from build123d import *

# Parameters (mm, degrees)
SKETCH1_W           = 24.7
SKETCH1_H           = 6.85
SKETCH1_R           = 1.4
BOSS_EXTRUDE1_DEPTH = 0.8
CHAMFER1_SIZE       = 1
SKETCH2_R           = 2
SKETCH2_R_2         = 1.4
BOSS_EXTRUDE2_DEPTH = 0.01


with BuildPart() as part:
    # Sketch1 → Boss-Extrude1 (new body, symmetric)
    with BuildSketch(Plane(origin=(0, 0, 0), x_dir=(1, 0, 0), z_dir=(0, 1, 0))):
        Rectangle(SKETCH1_W, SKETCH1_H)
        with Locations((-2.5, 0)):
            Circle(SKETCH1_R, mode=Mode.SUBTRACT)
        with Locations((2.5, 0)):
            Circle(SKETCH1_R, mode=Mode.SUBTRACT)
        with BuildLine():
            Line((-10.2, 1.25), (-6.8, 1.25))
            ThreePointArc((-6.8, 1.25), (-5.55, 0), (-6.8, -1.25))
            Line((-6.8, -1.25), (-10.2, -1.25))
            ThreePointArc((-10.2, -1.25), (-11.45, 0), (-10.2, 1.25))
        make_face(mode=Mode.SUBTRACT)
        with BuildLine():
            Line((10.2, 1.25), (6.8, 1.25))
            ThreePointArc((6.8, 1.25), (5.55, 0), (6.8, -1.25))
            Line((6.8, -1.25), (10.2, -1.25))
            ThreePointArc((10.2, -1.25), (11.45, 0), (10.2, 1.25))
        make_face(mode=Mode.SUBTRACT)
    extrude(amount=BOSS_EXTRUDE1_DEPTH, both=True)

    # Chamfer1
    chamfer1_edges = [part.edges().sort_by_distance(p)[0] for p in [
        (12.35, 0, 3.425),
        (-12.35, 0, 3.425),
        (-12.35, 0, -3.425),
        (12.35, 0, -3.425),
    ]]
    chamfer(chamfer1_edges, length=CHAMFER1_SIZE)

    # Sketch2 → Boss-Extrude2 (add)
    with BuildSketch(Plane(origin=(0, 0.8, 0), x_dir=(1, 0, 0), z_dir=(0, 1, 0))):
        with Locations((-2.5, 0)):
            Circle(SKETCH2_R)
        with Locations((-2.5, 0)):
            Circle(SKETCH2_R_2, mode=Mode.SUBTRACT)
        with Locations((2.5, 0)):
            Circle(SKETCH2_R)
        with Locations((2.5, 0)):
            Circle(SKETCH2_R_2, mode=Mode.SUBTRACT)
    boss_extrude2 = extrude(amount=BOSS_EXTRUDE2_DEPTH)

    # Mirror1: Boss-Extrude2 across plane
    add(boss_extrude2.mirror(Plane.ZX))


solid = part.part
Can you work these out from the model? Positions are in its coordinate system, mm. A direction names the side the tool comes from. Round coordinates to 2 decimals unless told otherwise and drop trailing zeros. Order: outer loops, then holes, each group sorted by start corner. A loop starts at its lowest first (then second) coordinate and runs counter-clockwise, first axis right, second up. Notation, with made-up numbers: (-17.5, 63.5) -> (-0.5, 63.5) arc R14 cw to (-0.5, 70.5) -> close; hole circle Ø1 at (29.25, 19). An arc over 180 degrees is marked (long way). Write each question's results on one line, items separated by ' | '. Start each with the question number.
Item 1: Thinking about a two-plate mould opening in X: for faces 3 (the flat face through (-1, 0.81, 1)), 4 (the flat face through (11.843, -0.011, 2.932)), 5 (the flat face through (-11.843, 0.011, -2.932)), 6 (the flat face through (-9, 0, -1.25)), which applies, +X half, -X half, draft (parallel to the pull), parting line (faces both ways), or undercut?
Item 2: If we section it at D-D, the plane x = 2.5: Write out the boundary of the cut face in (y, z) (3 decimals), then the cut area to 3 significant figures.
Item 3: Please list where these lines run through material, in increasing order: L1, parallel to X at y = 0.1, z = 0; L2, parallel to Z at x = 7.5, y = 0 (3 decimals); L3, parallel to Z at x = 2.5, y = 0 (3 decimals).
Item 4: Will this pin go through, and if not, where does the flat tip stop? pin 1 (3 mm diameter, centred on x = -2.5, z = 0, fed in from -Y).
Item 5: If we section it at A-A, the plane x = -8: Write out the boundary of the cut face in (y, z) (3 decimals).
Item 6: Which directions (+Z, -Z, +X, -X, +Y, -Y) give clear straight access to the entire face, cutting with the end or side of a thin tool? Please do faces 1 (the flat face through (0, 0, -3.425)), 2 (the cylindrical face through (-5.55, 0.01, -0.03)).
Item 7: If we section it at C-C, the plane z = -1: State how many separate pieces and enclosed holes the cut face has, then the cut area to 3 significant figures.
Item 8: If we section it at B-B, the plane y = -0.5: Write out the boundary of the cut face in (x, z) (3 decimals), then the cut area to 3 significant figures.
Results:
1) face 3: draft | face 4: +X half | face 5: -X half | face 6: undercut
2) outline: (-0.81, -2) -> (-0.8, -2) -> (-0.8, -3.425) -> (0.8, -3.425) -> (0.8, -2) -> (0.81, -2) -> (0.81, -1.4) -> (-0.81, -1.4) -> close; (-0.81, 1.4) -> (0.81, 1.4) -> (0.81, 2) -> (0.8, 2) -> (0.8, 3.425) -> (-0.8, 3.425) -> (-0.8, 2) -> (-0.81, 2) -> close | area: 6.50 mm2
3) L1: x = -12.35 to -11.45, -5.55 to -3.9, -1.1 to 1.1, 3.9 to 5.55, 11.45 to 12.35 | L2: z = -3.425 to -1.25, 1.25 to 3.425 | L3: z = -3.425 to -1.4, 1.4 to 3.425
4) pin 1: stops at y = -0.81
5) outline: (-0.8, -3.425) -> (0.8, -3.425) -> (0.8, -1.25) -> (-0.8, -1.25) -> close; (-0.8, 1.25) -> (0.8, 1.25) -> (0.8, 3.425) -> (-0.8, 3.425) -> close
6) face 1: -Z, +X, -X, +Y, -Y | face 2: +Y, -Y
7) separate pieces: 5 | enclosed holes: 0 | area: 17.6 mm2
8) outline: (-12.35, -2.425) -> (-11.35, -3.425) -> (11.35, -3.425) -> (12.35, -2.425) -> (12.35, 2.425) -> (11.35, 3.425) -> (-11.35, 3.425) -> (-12.35, 2.425) -> close; hole (-10.2, -1.25) -> (-6.8, -1.25) arc R1.25 ccw to (-6.8, 1.25) -> (-10.2, 1.25) arc R1.25 ccw to start; hole circle Ø2.8 at (-2.5, 0); hole circle Ø2.8 at (2.5, 0); hole (6.8, -1.25) -> (10.2, -1.25) arc R1.25 ccw to (10.2, 1.25) -> (6.8, 1.25) arc R1.25 ccw to start | area: 128 mm2
